Geometry: final body of the model. Coordinates: model frame, mm. Face numbers are marked on the shaded views. A direction names the side the tool comes from. Round coordinates to 2 decimals unless told otherwise and drop trailing zeros. Order: outer loops, then holes, each group sorted by start corner. A loop starts at its lowest first (then second) coordinate and runs counter-clockwise, first axis right, second up. Notation, with made-up numbers: (34, 66) - (74, 66) arc R24 ccw to (74, 82) - close; hole circle Ø6 at (-37, 72). An arc over 180 degrees is marked (long way). Put each result on its own line as item: value. Start each with the question number.
(1) Pin query (flat end, axial travel): P1, Ø16, axis at x = -52, y = 22.5, coming from the -Z side; P2, Ø8, axis at x = -52, y = 22.5, coming from the +Z side. Return the tip coordinate at first contact, or that it passes through.
(2) Section A-A (x = -52). Output: boundary loops of the cut face in (y, z), and give its area (3 significant figures).
(3) Access query for the marked faces 5 and 6. Directions: +Z, -Z, +X, -X, +Y, -Y. A direction counts if a zero-diameter tool reaches every point of the face in a straight line with its end or side. Return the directions, or none.
(4) Section B-B (y = 22.5). Output: boundary loops of the cut face in (x, z), and give its area (3 significant figures).
(5) Section C-C (x = -20.5). Output: boundary loops of the cut face in (y, z), and give its area (3 significant figures).
(6) Material intervals for L1, parallel to X at y = 42, z = -130; L2, parallel to Z at x = -84.5, y = 9.5; L3, parallel to Y at x = -15, z = -44, sorted ascending. Write a range as [from, to].
(7) Section D-D (y = 43). Output: boundary loops of the cut face in (x, z).
(8) Pull-direction query (X, two-part tool) for the marked faces 1, 2, 3 and 4; classes: released by +X, released by -X, zero draft, split by the parting line, or undercut.
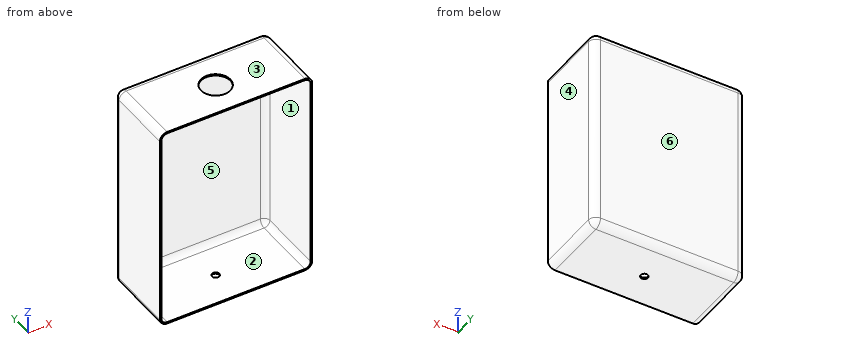
Autodesk Inventor part; units mm, degrees
ref_plane "YZ Plane" through (0, 0, 0) normal (1, 0, 0) x (0, 1, 0)
ref_plane "XZ Plane" through (0, 0, 0) normal (0, 1, 0) x (-1, 0, 0)
ref_plane "XY Plane" through (0, 0, 0) normal (0, 0, 1) x (1, 0, 0)
sketch "Sketch1" plane through (0, 0, 0) normal (0, 1, 0) x (-1, 0, 0)
  line L0 (0, 0) -> (104, 0)
  line L1 (104, 0) -> (104, -142)
  line L2 (104, -142) -> (0, -142)
  line L3 (0, -142) -> (0, 0)
  dimension "d0" = 142
  dimension "d1" = 104
extrude "Extrusion1" add sketch "Sketch1" along normal blind 50
fillet "Fillet1" radius 5 8 edges at (-104, 50, -71) (-52, 50, 0) (-52, 50, -142) (0, 50, -71) (0, 25, 0) (0, 25, -142) (-104, 25, 0) (-104, 25, -142)
shell "Shell1" thickness 1 removed faces 1 at (-34.6667, 0, -93)
sketch "Sketch2" plane through (-99, 0, 0) normal (0, 0, 1) x (1, 0, 0)
  line L0 (94, 45) -> (94, 0)
  line L1 (0, 45) -> (94, 45)
  line L2 (0, 0) -> (0, 45)
  line L3 (0, 0) -> (94, 0)
  circle A0 centre (47, 22.5) radius 10
  point P0 (99, 0)
  dimension "d6" = 20
extrude "Extrusion2" cut sketch "Sketch2" against normal blind 50 contours A0
sketch "Sketch3" plane through (-5, 0, -142) normal (0, 0, -1) x (-1, 0, 0)
  line L0 (0, 0) -> (0, 45)
  line L1 (0, 0) -> (94, 0)
  line L2 (94, 45) -> (94, 0)
  line L3 (0, 45) -> (94, 45)
  circle A0 centre (47, 22.5) radius 2.5
  point P0 (-5, 0)
  dimension "d9" = 5
extrude "Extrusion3" cut sketch "Sketch3" against normal blind 50 contours A0
properties part number "aja arduino 2"
Checks:
1. P1: stops at z = -142
1. P2: stops at z = -141
2. outline: (0, -142) - (20, -142) - (20, -141) - (0, -141) - close; (0, -1) - (12.5, -1) - (12.5, 0) - (0, 0) - close; (25, -142) - (45, -142) arc R5 ccw to (50, -137) - (50, -5) arc R5 ccw to (45, 0) - (32.5, 0) - (32.5, -1) - (45, -1) arc R4 cw to (49, -5) - (49, -137) arc R4 cw to (45, -141) - (25, -141) - close
2. area: 211 mm²
3. face 5: -Y
3. face 6: +Z, -Z, +X, -X, +Y
4. outline: (-104, -137) arc R5 ccw to (-99, -142) - (-54.5, -142) - (-54.5, -141) - (-99, -141) arc R4 cw to (-103, -137) - (-103, -5) arc R4 cw to (-99, -1) - (-62, -1) - (-62, 0) - (-99, 0) arc R5 ccw to (-104, -5) - close; (-49.5, -142) - (-5, -142) arc R5 ccw to (0, -137) - (0, -5) arc R5 ccw to (-5, 0) - (-42, 0) - (-42, -1) - (-5, -1) arc R4 cw to (-1, -5) - (-1, -137) arc R4 cw to (-5, -141) - (-49.5, -141) - close
4. area: 455 mm²
5. outline: (0, -142) - (45, -142) arc R5 ccw to (50, -137) - (50, -5) arc R5 ccw to (45, 0) - (0, 0) - (0, -1) - (45, -1) arc R4 cw to (49, -5) - (49, -137) arc R4 cw to (45, -141) - (0, -141) - close
5. area: 236 mm²
6. L1: x = [-104, -103], [-1, 0]
6. L2: z = [-142, -141], [-1, 0]
6. L3: y = [49, 50]
7. outline: (-104, -137) arc R5 ccw to (-99, -142) - (-5, -142) arc R5 ccw to (0, -137) - (0, -5) arc R5 ccw to (-5, 0) - (-99, 0) arc R5 ccw to (-104, -5) - close; hole (-103, -137) arc R4 ccw to (-99, -141) - (-5, -141) arc R4 ccw to (-1, -137) - (-1, -5) arc R4 ccw to (-5, -1) - (-99, -1) arc R4 ccw to (-103, -5) - close
8. face 1: undercut
8. face 2: undercut
8. face 3: zero draft
8. face 4: released by +X
